Input: part model. Units: mm. Frame: model coordinates. Round coordinates to 2 decimals unless told otherwise and drop trailing zeros. Write each loop counter-clockwise with the first axis right and the second up, starting at its lowest first coordinate (ties: lowest second). Pieces come first, ordered by that corner, then holes. Notation, with made-up numbers: M 30,77.25 L 84,77.25 A24 ccw 84,95.25 Z; hole C 66.25,88 d5. An arc over 180 degrees is marked long. Answer as CSV lines item,"result". Start each with the question number.
Autodesk Inventor part; units mm, degrees
ref_plane "YZ Plane" through (0, 0, 0) normal (1, 0, 0) x (0, 1, 0)
ref_plane "XZ Plane" through (0, 0, 0) normal (0, 1, 0) x (-1, 0, 0)
ref_plane "XY Plane" through (0, 0, 0) normal (0, 0, 1) x (1, 0, 0)
sketch "Sketch1" plane through (0, 0, 0) normal (0, 1, 0) x (-1, 0, 0)
  point P0 (0, 0)
sketch "Sketch2" plane through (0, 0, 0) normal (0, 1, 0) x (-1, 0, 0)
  circle A0 centre (0, 0) radius 10 construction
  arc A1 (5.0714, -10.8757) -> (5.0714, 10.8757) centre (0, 0) ccw
  line L0 (5.0714, 10.8757) -> (5.0714, -10.8757) construction
  line L1 (5.0714, -10.8757) -> (92.8296, -10.8757)
  line L2 (5.0714, -10.8757) -> (92.8296, -10.8757) construction
  line L3 (80.2714, 10.8757) -> (92.8296, -10.8757)
  line L4 (80.2714, 10.8757) -> (5.0714, 10.8757)
  dimension "d0" = 20
  dimension "d2" = 2
  dimension "d3" = 130
  dimension "d5" = 0
  dimension "d14" = 75.2
  dimension "d15" = 12.5582
extrude "Extrusion1" add sketch "Sketch2" along normal blind 10
sketch "Sketch3" plane through (0, 10, 0) normal (0, 1, 0) x (1, 0, 0)
  line L0 (-80.2714, -10.8757) -> (-92.8296, 10.8757)
  line L1 (-80.2714, -10.8757) -> (-61.4714, -43.4382)
  arc A0 (-5.0714, 10.8757) -> (-5.0714, -10.8757) centre (0, 0) ccw
  line L2 (-61.4714, -43.4382) -> (-5.0714, -10.8757)
  line L3 (-80.2714, -10.8757) -> (-5.0714, -10.8757)
  line L4 (-80.2714, -10.8757) -> (-5.0714, -10.8757)
  point P0 (-104.4015, 68.9975)
  point P1 (-92.8296, 10.8757)
extrude "Extrusion2" add sketch "Sketch3" against normal blind 10
sketch "Sketch4" plane through (0, 10, 0) normal (0, 1, 0) x (1, 0, 0)
  circle A0 centre (-54.7759, -15.0352) radius 1.25
  circle A1 centre (-37.4554, -5.0352) radius 1.25
  line L0 (-54.7759, -15.0352) -> (-37.4554, -5.0352) construction
  line L1 (-61.4714, -43.4382) -> (-5.0714, -10.8757) construction
  line L2 (-92.8296, 10.8757) -> (-61.4714, -43.4382) construction
  point P0 (0, 0)
  dimension "d16" = 2.5
  dimension "d17" = 2.5
  dimension "d18" = 20
  dimension "d19" = 20
  dimension "d20" = 21.25
extrude "Extrusion3" cut sketch "Sketch4" along normal through all both and the other way through all
properties part number "flipper-hug-left-2"
Item 1: Line query: line 1 (X direction, y = 0.5, z = 14.5); line 2 (Z direction, x = -10.5, y = 6); line 3 (Z direction, x = -35.5, y = 9.5). Output: solid intervals per line, ascending. Write a range as [from, to].
Item 2: Draft query along Z for faces 1 (the face through (-33.666, 5.07, 27.385)), 2 (the face through (-48, 0, 11)), 3 (the face through (-55.047, 5.07, 16.255)), 4 (the face through (-12, 5, 0)). Return one class per face: +Z half, -Z half, draft (parallel to the pull), parting line (faces both ways), or undercut.
Item 3: Pin query (flat end, axial travel): pin 1 Ø1.5 at (y, z) = (1.5, -4) entering from -X; pin 2 Ø3 at (y, z) = (3, -1.5) entering from -X. Return the tip coordinate at first contact, or that it passes through.
Item 4: Cut plane A-A, the plane y = 7. Return loops of the section in (x, z), plus the area to 3 significant figures.
Item 5: Cut plane C-C, the plane z = 28.5. Return loops of the section in (x, y).
Item 6: Cut plane B-B, the plane x = -9.5. Return loops of the section in (y, z), plus the area to 3 significant figures.
Item 7: Cut plane D-D, the plane x = -31. Return loops of the section in (y, z), plus the area to 3 significant figures.
Results list:
1,line 1,"[-78.18, -55.91], [-53.65, -11.35]"
1,line 2,"[-10.88, -5.81], [5.81, 14.01]"
1,line 3,"[-10.88, 28.44]"
2,face 1,"+Z half"
2,face 2,"draft"
2,face 3,"undercut"
2,face 4,"undercut"
3,pin 1,"x = -89.29"
3,pin 2,"x = -88.28"
4,outline,"M -92.83,-10.88 L -5.07,-10.88 A12 cw -5.07,10.88 L -61.47,43.44 Z; hole C -54.78,15.04 d2.5; hole C -37.46,5.04 d2.5"
4,area,"2,880 mm²"
5,outline,"M -70.1,0 L -35.6,0 L -35.6,10 L -70.1,10 Z"
6,outline,"M 0,-10.88 L 10,-10.88 L 10,-7.33 L 0,-7.33 Z; M 0,7.33 L 10,7.33 L 10,13.43 L 0,13.43 Z"
6,area,"96.5 mm²"
7,outline,"M 0,-10.88 L 10,-10.88 L 10,25.85 L 0,25.85 Z"
7,area,"367 mm²"
